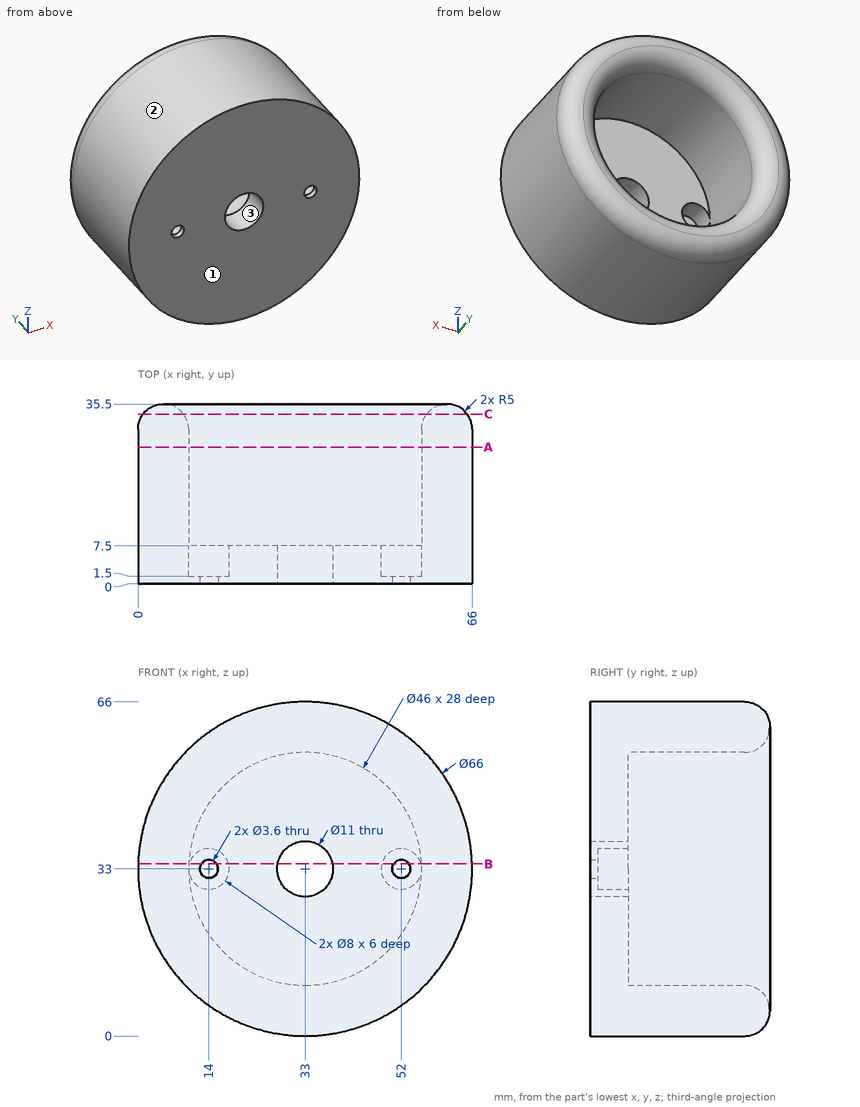
Verification items for this drawing (mm, ordinates from the low corner). Coordinates: 2 decimals unless noted, no trailing zeros. Write each loop counter-clockwise with the first axis right and the second up, starting at its lowest first coordinate (ties: lowest second). Pieces come first, ordered by that corner, then holes. Notation, with made-up numbers: (-12, 17) - (-5, 17) arc R23 cw to (-5, 42) - close; hole circle Ø7 at (20.25, -21). An arc over 180 degrees is marked (long way). One line per question, with ' | ' between items.
Item 1: Sectioned sample at A-A on y = 27. Record the boundary of the cut face in (x, z).
Determined:
outline: circle Ø66 at (33, 33); hole circle Ø46 at (33, 33)
Item 2: Gauge pin test, flat ends, axial feed: P1, Ø3, axis at y = 20.5, z = 17, coming from the +X side; P2, Ø5, axis at x = 46, z = 37, coming from the +Y side; P3, Ø6, axis at x = 38, y = 6.5, coming from the +Z side. Record the tip position at first contact, or that the pin passes through.
Determined:
P1: stops at x = 62.64 | P2: stops at y = 7.5 | P3: stops at z = 65.94
Item 3: Sectioned sample at C-C on y = 33.5. Record the boundary of the cut face in (x, z), plus the area to 3 significant figures.
Determined:
outline: circle Ø64 at (33, 33); hole circle Ø48 at (33, 33) | area: 1,410 mm2
Item 4: Thickness scan on line 1 (X direction, y = 4.5, z = 33); line 2 (X direction, y = 1, z = 33); line 3 (X direction, y = 27.5, z = 16.5). Record the ranges inside material, lowest first. Write a range as [from, to].
Determined:
line 1: x = [0, 10], [18, 27.5], [38.5, 48], [56, 66] | line 2: x = [0, 12.2], [15.8, 27.5], [38.5, 50.2], [53.8, 66] | line 3: x = [4.42, 16.98], [49.02, 61.58]
Item 5: Sectioned sample at B-B on z = 34. Give the number of separate pieces and of enclosed holes in the cut face, plus the area to 3 significant figures.
Determined:
separate pieces: 4 | enclosed holes: 0 | area: 851 mm2
Item 6: Mould release check, pull along X, two halves, no side actions. Record for the marked faces 1, 2 and 3: pulls with the +X half, pulls with the -X half, needs draft (parallel to the pull), parting line crosses it, or undercut.
Determined:
face 1: needs draft | face 2: parting line crosses it | face 3: undercut
